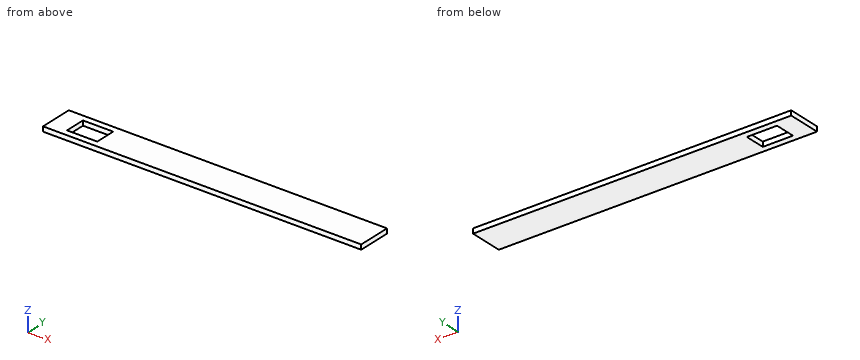
Autodesk Inventor part; units mm, degrees
ref_plane "YZ Plane" through (0, 0, 0) normal (1, 0, 0) x (0, 1, 0)
ref_plane "XZ Plane" through (0, 0, 0) normal (0, 1, 0) x (-1, 0, 0)
ref_plane "XY Plane" through (0, 0, 0) normal (0, 0, 1) x (1, 0, 0)
sketch "block" plane through (0, 0, 0) normal (0, 1, 0) x (-1, 0, 0)
  line L0 (0, 0) -> (-200, 0)
  line L1 (-200, 0) -> (-200, -250)
  line L2 (-200, -250) -> (0, -250)
  line L3 (0, -250) -> (0, 0)
  dimension "d31" = 200
  dimension "d32" = 250
extrude "ext_block" add sketch "block" against normal blind 24
shell "Shell2" thickness 3 removed faces 0
sketch "lines_base" plane through (0, 0, 0) normal (0, 1, 0) x (-1, 0, 0)
  line L0 (0, 0) -> (-200, 0)
  line L1 (-200, 0) -> (-200, -250)
  line L2 (-200, -250) -> (0, -250)
  line L3 (0, -250) -> (0, 0)
  circle A0 centre (-65, -60) radius 6
  circle A1 centre (-125, -80) radius 6
  circle A2 centre (-65, -60) radius 12.5
  circle A3 centre (-65, -60) radius 8.5
  circle A4 centre (-125, -80) radius 8.5
  circle A5 centre (-125, -80) radius 12.5
  circle A6 centre (-175, -125) radius 3
  line L4 (-175, -125) -> (-175, -209)
  line L5 (-175, -125) -> (-91, -125) construction
  circle A7 centre (-175, -139) radius 3
  circle A8 centre (-175, -153) radius 3
  circle A9 centre (-175, -167) radius 3
  circle A10 centre (-175, -181) radius 3
  circle A11 centre (-175, -195) radius 3
  circle A12 centre (-175, -209) radius 3
  circle A13 centre (-95, -185) radius 2.5
  circle A14 centre (-95, -185) radius 5
  point P0 (-200, -125)
  dimension "d0" = 200
  dimension "d1" = 250
  dimension "d2" = 12
  dimension "d3" = 12
  dimension "d4" = 25
  dimension "d5" = 17
  dimension "d6" = 17
  dimension "d7" = 25
  dimension "d8" = 75
  dimension "d9" = 80
  dimension "d10" = 65
  dimension "d11" = 60
  dimension "d12" = 6
  dimension "d13" = 84
  dimension "d14" = 90
  dimension "d15" = 25
  dimension "d16" = 125
  dimension "d19" = 14
  dimension "d24" = 5
  dimension "d25" = 10
  dimension "d26" = 65
  dimension "d27" = 95
extrude "holes" cut sketch "lines_base" against normal up to surface (3 mm away) contours A0 | A1 | A6 | A7 L4 | L4 A7 | A8 L4 | L4 A8 | A9 L4 | L4 A9 | A10 L4 | L4 A10 | A11 L4 | L4 A11 | A12 | A13
sketch "Sketch4" plane through (200, 0, -250) normal (0, 0, -1) x (-1, 0, 0)
  line L0 (188, -4) -> (169, -4)
  line L1 (169, -4) -> (169, -17)
  line L2 (169, -17) -> (188, -17)
  line L3 (188, -17) -> (188, -4)
  line L4 (0, 0) -> (200, 0)
  line L5 (200, 0) -> (200, -24)
  dimension "d40" = 19
  dimension "d41" = 13
  dimension "d42" = 4
  dimension "d43" = 12
extrude "pwr_button_hole" cut sketch "Sketch4" against normal up to surface (3 mm away)
ref_plane "Work Plane1" through (7, -21, -243) normal (0, 1, 0) x (1, 0, 0)
sketch "Sketch5" plane through (7, -21, -243) normal (0, 1, 0) x (1, 0, 0)
  line L0 (-20.9366, 21.7948) -> (229.9216, 21.7948)
  line L1 (229.9216, 21.7948) -> (229.9216, -260.9184)
  line L2 (229.9216, -260.9184) -> (-20.9366, -260.9184)
  line L3 (-20.9366, -260.9184) -> (-20.9366, 21.7948)
  point P0 (-7, -243)
extrude "back_cover_cut" cut sketch "Sketch5" against normal through all
sketch "Sketch9" plane through (3, -3, -247) normal (0, 0, 1) x (1, 0, 0)
  line L0 (-37.3239, 25.5636) -> (215.9348, 25.5636)
  line L1 (215.9348, 25.5636) -> (215.9348, -44.9988)
  line L2 (215.9348, -44.9988) -> (-37.3239, -44.9988)
  line L3 (-37.3239, -44.9988) -> (-37.3239, 25.5636)
  point P0 (-3, 3)
extrude "Extrusion8" cut sketch "Sketch9" along normal through all
properties part number "side_right" material "Glass"
Read the model definition and answer for the solid it produces. Units are mm, in the model's axes. Give positions to 0.01 mm unless a question says otherwise; leave off trailing zeros. Write each loop counter-clockwise with the first axis right and the second up, starting at its lowest first coordinate (ties: lowest second). Pieces come first, ordered by that corner, then holes. Notation, with made-up numbers: (5, -21) - (63, -21) arc R18 ccw to (63, 0) - close; hole circle Ø4 at (14, 69.5). An arc over 180 degrees is marked (long way). Return JSON: item names as keys, results as strings.
Q1. Consider line 1 along X through (y, z) = (-14.25, -249.2); line 2 along Y through (x, z) = (21, -248.65). Determine where each line is inside the solid, lowest interval first. Write a range as [from, to].
Reply:
{"line 1": "[0, 12], [31, 200]", "line 2": "[-21, -17], [-4, 0]"}
Q2. A cutting plane is placed at B-B, the plane z = -249.15. Determine the outline of the cut face in (x, y), and give its area (3 significant figures).
Reply:
{"outline": "(0, -21) - (200, -21) - (200, 0) - (0, 0) - close; hole (12, -17) - (31, -17) - (31, -4) - (12, -4) - close", "area": "3,950 mm²"}
Q3. Given P1, Ø1.5, axis at y = -13, z = -248.5, coming from the -X side, flat-ended and moving along its own axis, determine where the tip first touches the part or whether it passes through.
Reply:
{"P1": "x = 0"}
Q4. A cutting plane is placed at A-A, the plane y = -5.75. Determine the outline of the cut face in (x, z).
Reply:
{"outline": "(0, -250) - (12, -250) - (12, -247) - (0, -247) - close; (31, -250) - (200, -250) - (200, -247) - (31, -247) - close"}
